The listing builds one solid part. Answer for the finished solid, in the listing's coordinates (mm). Face numbers are marked on the shaded views. Round coordinates to 2 decimals unless told otherwise and drop trailing zeros. Loops run counter-clockwise (first coordinate to the right, second up) from the corner with the lowest first, then second, coordinate; pieces in that order, holes last. Notation, with made-up numbers: (72, 21.25) -> (119, 21.25) arc R24 ccw to (119, 54.25) -> close; hole circle Ø9 at (88, 15). An arc over 180 degrees is marked (long way). Answer in a Markdown table with one row per item. Add a question column.
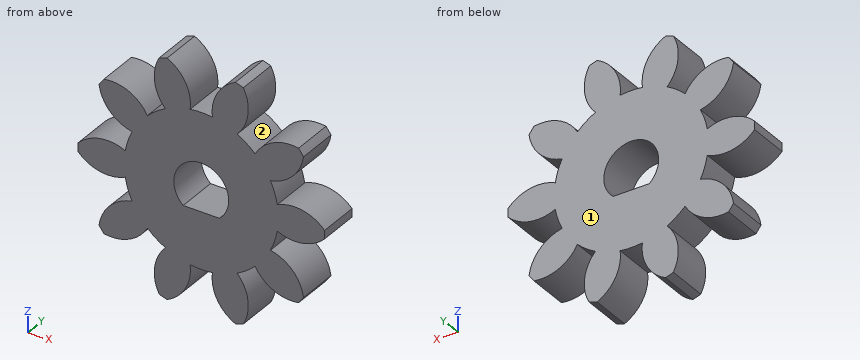
```python
from build123d import *

# Parameters (mm, degrees)
SKETCH1_R           = 9
BOSS_EXTRUDE1_DEPTH = 3
CUT_EXTRUDE1_DEPTH  = 4
CIRPATTERN1_COUNT   = 10
CUT_EXTRUDE5_DEPTH  = 4


with BuildPart() as part:
    # Sketch1 → Boss-Extrude1 (new body)
    with BuildSketch(Plane(origin=(0, 0, 0), x_dir=(1, 0, 0), z_dir=(0, 1, 0))):
        Circle(SKETCH1_R)
    extrude(amount=BOSS_EXTRUDE1_DEPTH)

    # Sketch2 → Cut-Extrude1 (cut, through all)
    with BuildSketch(Plane(origin=(0, 3, 0), x_dir=(1, 0, 0), z_dir=(0, 1, 0))):
        with BuildLine():
            ThreePointArc((-0.810569881, 5.566291536), (0, 5.625), (0.810569881, 5.566291536))
            ThreePointArc((0.810569881, 5.566291536), (1.152028564, 7.378729724), (2.489254397, 8.648908171))
            ThreePointArc((2.489254397, 8.648908171), (0, 9), (-2.489254397, 8.648908171))
            ThreePointArc((-2.489254397, 8.648908171), (-1.152028564, 7.378729724), (-0.810569881, 5.566291536))
        make_face()
    cut_extrude1 = extrude(amount=-CUT_EXTRUDE1_DEPTH, mode=Mode.SUBTRACT)

    # CirPattern1: Cut-Extrude1 ×10 about axis
    cirpattern1_axis = Axis((0, 0, 0), (0, 1, 0))
    for i in range(1, CIRPATTERN1_COUNT):
        add(cut_extrude1.rotate(cirpattern1_axis, i * 360 / CIRPATTERN1_COUNT), mode=Mode.SUBTRACT)

    # Sketch6 → Cut-Extrude5 (cut, through all)
    with BuildSketch(Plane(origin=(0, 3, 0), x_dir=(1, 0, 0), z_dir=(0, 1, 0))):
        with BuildLine():
            Line((1.322875656, 1.5), (-1.322875656, 1.5))
            ThreePointArc((-1.322875656, 1.5), (0, -2), (1.322875656, 1.5))
        make_face()
    extrude(amount=-CUT_EXTRUDE5_DEPTH, mode=Mode.SUBTRACT)


solid = part.part
```
Item 1: Section C-C, the plane z = 4.5 is taken. Write down the section's boundary in (x, y) (3 decimals).
Item 2: Consider L1, parallel to X at y = 1.85, z = 0; L2, parallel to X at y = 1.8, z = 4.25; L3, parallel to Z at x = -3, y = 2.15. Determine where each line is inside the solid, lowest interval first. Write a range as from..to.
Item 3: Section A-A, the plane x = 0 is taken. Write down the section's boundary in (y, z) (3 decimals).
Item 4: Section B-B, the plane z = 0 is taken. Write down the section's boundary in (x, y).
Item 5: The mould has two halves that part along X. Classify the marked faces 1 and 2: +X half, -X half, draft (parallel to the pull), parting line (faces both ways), or undercut.
Here are the results:
| question | item | result |
|---|---|---|
| 1 | outline | (-7.332, 0) -> (-4.25, 0) -> (-4.25, 3) -> (-7.332, 3) -> close; (-3.375, 0) -> (3.375, 0) -> (3.375, 3) -> (-3.375, 3) -> close; (4.25, 0) -> (7.332, 0) -> (7.332, 3) -> (4.25, 3) -> close |
| 2 | L1 | x = -9..-2, 2..9 |
| 2 | L2 | x = -7.24..-4.06, -3.68..3.68, 4.06..7.24 |
| 2 | L3 | z = -8.49..-5.49, -4.76..4.76, 5.49..8.49 |
| 3 | outline | (0, -5.625) -> (3, -5.625) -> (3, -1.5) -> (0, -1.5) -> close; (0, 2) -> (3, 2) -> (3, 5.625) -> (0, 5.625) -> close |
| 4 | outline | (-9, 0) -> (-2, 0) -> (-2, 3) -> (-9, 3) -> close; (2, 0) -> (9, 0) -> (9, 3) -> (2, 3) -> close |
| 5 | face 1 | draft |
| 5 | face 2 | undercut |
